```python
from build123d import *

# Parameters (mm, degrees)
F0_W      = 200
F0_H      = 200
F0_R      = 2
F1_DEPTH  = 10
F2_R      = 40
F2_R_2    = 38
F3_DEPTH  = 100
F7_SIZE   = 1
F8_SIZE   = 1
F10_R     = 4
F11_DEPTH = 80
F12_DEPTH = 25


with BuildPart() as f1:
    # F0 (on Top) → F1 (new body)
    with BuildSketch(Plane.XY):
        Rectangle(F0_W, F0_H)
        with Locations((-53.033009, -53.033009)):
            Circle(F0_R, mode=Mode.SUBTRACT)
        with Locations((0, -75)):
            Circle(F0_R, mode=Mode.SUBTRACT)
        with Locations((53.033009, -53.033009)):
            Circle(F0_R, mode=Mode.SUBTRACT)
        with Locations((-75, 0)):
            Circle(F0_R, mode=Mode.SUBTRACT)
        with Locations((-53.033009, 53.033009)):
            Circle(F0_R, mode=Mode.SUBTRACT)
        with Locations((75, 0)):
            Circle(F0_R, mode=Mode.SUBTRACT)
        with Locations((0, 75)):
            Circle(F0_R, mode=Mode.SUBTRACT)
        with Locations((53.033009, 53.033009)):
            Circle(F0_R, mode=Mode.SUBTRACT)
    extrude(amount=-F1_DEPTH)

    # F2 (on face) → F3 (join)
    with BuildSketch(Plane.XY):
        Circle(F2_R)
        Circle(F2_R_2, mode=Mode.SUBTRACT)
    extrude(amount=F3_DEPTH)

    # F5 (on Front) → F6 (revolve)
    with BuildSketch(Plane.XZ):
        Polygon((0, 52), (0, 50), (22, 50), (22, 100), (40, 100), (40, 102), (20, 102), (20, 52), align=None)
    revolve(axis=Axis((0, 0, 75.148744), (0, 0, 1)))

    # F7
    f7_edges = [f1.edges().sort_by_distance(p)[0] for p in [
        (-40, 0, 0),
        (40, 0, 51),
        (-40, 0, 102),
    ]]
    chamfer(f7_edges, length=F7_SIZE)

    # F8
    f8_edges = [f1.edges().sort_by_distance(p)[0] for p in [
        (-20, 0, 102),
    ]]
    chamfer(f8_edges, length=F8_SIZE)

    # F10 (on offset) → F11 (cut)
    with BuildSketch(Plane.XZ.offset(40)):
        with Locations((0, 77)):
            Circle(F10_R)
    extrude(amount=-F11_DEPTH, mode=Mode.SUBTRACT)

    # F0 (on Top) → F12 (cut)
    with BuildSketch(Plane.XY):
        with Locations((0, 75)):
            Circle(F0_R)
    extrude(amount=-F12_DEPTH, mode=Mode.SUBTRACT)


solid = f1.part
```
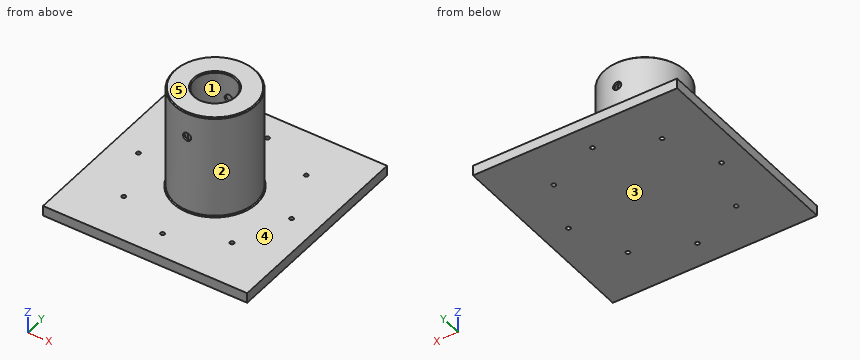
The model under review builds one solid part; all positions refer to its coordinate system, in mm. Face numbers are marked on the shaded views. A direction names the side the tool comes from. Give positions to 0.01 mm unless a question says otherwise; leave off trailing zeros. Write each loop counter-clockwise with the first axis right and the second up, starting at its lowest first coordinate (ties: lowest second). Pieces come first, ordered by that corner, then holes. Notation, with made-up numbers: M 10.25,-39.5 L 20.25,-39.5 A23 cw 20.25,-18.5 Z; hole C 86.5,1.5 d9. An arc over 180 degrees is marked long. Answer in a Markdown table with one row per item.
Item 1: Add section A-A on z = 83.5. Give the boundary of the cut face in (x, y), plus the area to 3 significant figures.
Check sheet entries:
| item | result |
|---|---|
| outline | C 0,0 d80; C 0,0 d44; hole C 0,0 d76; hole C 0,0 d40 |
| area | 754 mm2 |
Item 2: Draft analysis for pull direction Y (two halves, no side actions). For the marked faces 1, 2 and 3, state which applies: +Y half, -Y half, draft (parallel to the pull), parting line (faces both ways), or undercut.
Check sheet entries:
| item | result |
|---|---|
| face 1 | undercut |
| face 2 | parting line |
| face 3 | draft |
Item 3: For P1, Ø2, axis at x = 7, z = 9, coming from the -Y side; P2, Ø5, axis at x = -63, y = -59.5, coming from the +Z side; P3, Ø9, axis at x = 0, z = 77, coming from the -Y side; P4, Ø4.5, axis at x = -53.03, y = 53.03, coming from the -Z side, all flat-tipped, find the tip position at first contact; note any pin that passes through.
Check sheet entries:
| item | result |
|---|---|
| P1 | y = -39.55 |
| P2 | z = 0 |
| P3 | y = -40 |
| P4 | z = -10 |
Item 4: Tool access review of the marked faces 4 and 5: name each direction out of +Z, -Z, +X, -X, +Y, -Y from which nothing blocks a thin tool from reaching the whole face with its end or side.
Check sheet entries:
| item | result |
|---|---|
| face 4 | +Z |
| face 5 | +Z, +X, -X, +Y, -Y |
Item 5: For line 1 along Z through (x, y) = (0, -21); line 2 along Y through (x, z) = (0, -7.25); line 3 along X through (y, z) = (6.5, 69.5), list the stretches that pass through material, from the lowest coordinate up.
Check sheet entries:
| item | result |
|---|---|
| line 1 | -10 to 0, 50 to 73, 81 to 102 |
| line 2 | -100 to -77, -73 to 73, 77 to 100 |
| line 3 | -39.47 to -37.44, -21.02 to -18.91, 18.91 to 21.02, 37.44 to 39.47 |
Item 6: Add section B-B on x = -80. Give the boundary of the cut face in (y, z).
Check sheet entries:
| item | result |
|---|---|
| outline | M -100,-10 L 100,-10 L 100,0 L -100,0 Z |
Item 7: Add section C-C on z = 39. Give the boundary of the cut face in (x, y).
Check sheet entries:
| item | result |
|---|---|
| outline | C 0,0 d80; hole C 0,0 d76 |
